```python
from build123d import *

# Parameters (mm, degrees)
SZKIC1_W                    = 80
SZKIC1_H                    = 35
SZKIC1_R                    = 1.5
DODANIE_WYCI_GNI_CIE1_DEPTH = 4
SZKIC2_W                    = 70
SZKIC2_H                    = 23
DODANIE_WYCI_GNI_CIE2_DEPTH = 6


with BuildPart() as part:
    # Szkic1 → Dodanie-wyciągnięcie1 (new body)
    with BuildSketch(Plane(origin=(0, 0, 0), x_dir=(1, 0, 0), z_dir=(0, 1, 0))):
        Rectangle(SZKIC1_W, SZKIC1_H)
        with Locations((-37.5, 15)):
            Circle(SZKIC1_R, mode=Mode.SUBTRACT)
        with Locations((-37.5, -15)):
            Circle(SZKIC1_R, mode=Mode.SUBTRACT)
        with Locations((37.5, -15)):
            Circle(SZKIC1_R, mode=Mode.SUBTRACT)
        with Locations((37.5, 15)):
            Circle(SZKIC1_R, mode=Mode.SUBTRACT)
    extrude(amount=DODANIE_WYCI_GNI_CIE1_DEPTH)

    # Szkic2 → Dodanie-wyciągnięcie2 (add)
    with BuildSketch(Plane(origin=(0, 4, 0), x_dir=(1, 0, 0), z_dir=(0, 1, 0))):
        Rectangle(SZKIC2_W, SZKIC2_H)
    extrude(amount=DODANIE_WYCI_GNI_CIE2_DEPTH)


solid = part.part
```
Here's how the part is built. I have some questions about the finished solid (model axes, mm). A direction names the side the tool comes from. Round coordinates to 2 decimals unless told otherwise and drop trailing zeros. Loops run counter-clockwise (first coordinate to the right, second up) from the corner with the lowest first, then second, coordinate; pieces in that order, holes last.
1. Suppose I cut it at D-D, the plane x = 3. Please give me the cut outline in (y, z), and give its area (3 significant figures).
Answers:
outline: (0, -17.5) - (4, -17.5) - (4, -11.5) - (10, -11.5) - (10, 11.5) - (4, 11.5) - (4, 17.5) - (0, 17.5) - close
area: 278 mm2
2. If I drill on probe 1 along Z at (x, y) = (-37.5, 2.85); probe 2 along X at (y, z) = (1.95, -15); probe 3 along Z at (x, y) = (-34.5, 4.5), over which ranges is the centre line in solid material (lowest first)?
Answers:
probe 1: z = -17.5 to -16.5, -13.5 to 13.5, 16.5 to 17.5
probe 2: x = -40 to -39, -36 to 36, 39 to 40
probe 3: z = -11.5 to 11.5
3. Suppose I cut it at A-A, the plane z = 15. Please give me the cut outline in (x, y), and give its area (3 significant figures).
Answers:
outline: (-40, 0) - (-39, 0) - (-39, 4) - (-40, 4) - close; (-36, 0) - (36, 0) - (36, 4) - (-36, 4) - close; (39, 0) - (40, 0) - (40, 4) - (39, 4) - close
area: 296 mm2
4. Suppose I cut it at B-B, the plane x = -37.5. Please give me the cut outline in (y, z), and give its area (3 significant figures).
Answers:
outline: (0, -17.5) - (4, -17.5) - (4, -16.5) - (0, -16.5) - close; (0, -13.5) - (4, -13.5) - (4, 13.5) - (0, 13.5) - close; (0, 16.5) - (4, 16.5) - (4, 17.5) - (0, 17.5) - close
area: 116 mm2
5. For faces 1 (the face through (-35, 7, 0)), 2 (the face through (0, 7, 11.5)), 3 (the face through (35, 7, 0)), which set-ups out of +Z, -Z, +X, -X, +Y, -Y let a thin tool reach every point of the face, with its end or its side?
Answers:
face 1: +Z, -Z, -X, +Y
face 2: +Z, +X, -X, +Y
face 3: +Z, -Z, +X, +Y
6. Thinking about a two-plate mould opening in Z: for faces 4 (the face through (36.3, 2, -14.1)), 5 (the face through (40, 2, 0)), 6 (the face through (-1, 2, -17.5)), which applies, released by +Z, released by -Z, zero draft, split by the parting line, or undercut?
Answers:
face 4: undercut
face 5: zero draft
face 6: released by -Z
7. Will these pins go through, and if not, where does the flat tip stop? pin 1 (4 mm diameter, centred on x = -37.5, z = 15, fed in from +Y); pin 2 (1.8 mm diameter, centred on y = 7.5, z = 2, fed in from +X); pin 3 (1.8 mm diameter, centred on y = 8.5, z = 1, fed in from -X); pin 4 (4 mm diameter, centred on x = 17, z = -13.5, fed in from -Y).
Answers:
pin 1: stops at y = 4
pin 2: stops at x = 35
pin 3: stops at x = -35
pin 4: stops at y = 0
8. Suppose I cut it at C-C, the plane z = -4. Please give me the cut outline in (x, y), and give its area (3 significant figures).
Answers:
outline: (-40, 0) - (40, 0) - (40, 4) - (35, 4) - (35, 10) - (-35, 10) - (-35, 4) - (-40, 4) - close
area: 740 mm2
